Verification items for the finished model (mm, model axes). Give positions to 0.01 mm unless a question says otherwise; leave off trailing zeros. Order: outer loops, then holes, each group sorted by start corner. A loop starts at its lowest first (then second) coordinate and runs counter-clockwise, first axis right, second up.
(1) Sectioned sample at B-B on x = 20.5. Record the cut outline in (y, z), plus the area to 3 significant figures.
(2) Scan lines: L1, parallel to X at y = 1.7, z = -16; L2, parallel to Z at x = 57, y = -0.4; L3, parallel to X at y = -1.5, z = -10. Record each from-to range of solid material in increasing order.
(3) Gauge pin test, flat ends, axial feed: pin 1 (3 mm diameter, centred on y = 2, z = -9.5, fed in from +X); pin 2 (1.5 mm diameter, centred on y = 0.5, z = -13.5, fed in from +X); pin 3 (2.5 mm diameter, centred on y = 0.5, z = 15.5, fed in from +X); pin 4 (1.5 mm diameter, centred on y = 0.5, z = 17, fed in from -X). Record the tip position at first contact, or that the pin passes through.
(4) Sectioned sample at A-A on z = 5.5. Record the cut outline in (x, y), plus the area to 3 significant figures.
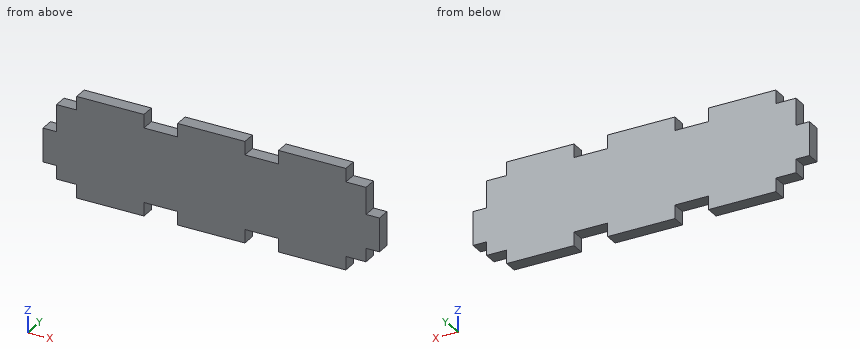
```python
from build123d import *

# Parameters (mm, degrees)
SKETCH1_W           = 127
SKETCH1_H           = 38.1
BOSS_EXTRUDE1_DEPTH = 2.54
SKETCH2_W           = 5.08
SKETCH2_H           = 10.16
SKETCH2_H_2         = 15.24
CUT_EXTRUDE1_DEPTH  = 5.08
SKETCH3_W           = 12.7
SKETCH3_H           = 5.08
CUT_EXTRUDE2_DEPTH  = 5.08
SKETCH4_W           = 12.7
SKETCH4_H           = 5.08
CUT_EXTRUDE4_DEPTH  = 5.08
LPATTERN1_COUNT     = 2
LPATTERN1_PITCH     = 38.1
SKETCH7_W           = 116.84
SKETCH7_H           = 5.08
CUT_EXTRUDE7_DEPTH  = 5.08
SKETCH8_W           = 25.4
SKETCH8_H           = 5.08
BOSS_EXTRUDE2_DEPTH = 5.08


with BuildPart() as part:
    # Sketch1 → Boss-Extrude1 (new body, symmetric)
    with BuildSketch(Plane(origin=(0, 0, 0), x_dir=(1, 0, 0), z_dir=(0, 1, 0))):
        Rectangle(SKETCH1_W, SKETCH1_H)
    extrude(amount=BOSS_EXTRUDE1_DEPTH, both=True)

    # Sketch2 → Cut-Extrude1 (cut)
    with BuildSketch(Plane(origin=(0, 2.54, 0), x_dir=(1, 0, 0), z_dir=(0, 1, 0))):
        with Locations((-60.96, 13.97)):
            Rectangle(SKETCH2_W, SKETCH2_H)
        with Locations((-60.96, -11.43)):
            Rectangle(SKETCH2_W, SKETCH2_H_2)
    cut_extrude1 = extrude(amount=-CUT_EXTRUDE1_DEPTH, mode=Mode.SUBTRACT)

    # Mirror1: Cut-Extrude1 across plane
    add(cut_extrude1.mirror(Plane(origin=(0, 0, 0), x_dir=(0, 0, 1), z_dir=(1, 0, 0))), mode=Mode.SUBTRACT)

    # Sketch3 → Cut-Extrude2 (cut)
    with BuildSketch(Plane(origin=(0, 2.54, 0), x_dir=(1, 0, 0), z_dir=(0, 1, 0))):
        with Locations((-57.15, -16.51)):
            Rectangle(SKETCH3_W, SKETCH3_H)
    cut_extrude2 = extrude(amount=-CUT_EXTRUDE2_DEPTH, mode=Mode.SUBTRACT)

    # Mirror2: Cut-Extrude2 across plane
    add(cut_extrude2.mirror(Plane(origin=(0, 0, 0), x_dir=(0, 0, 1), z_dir=(1, 0, 0))), mode=Mode.SUBTRACT)

    # Sketch4 → Cut-Extrude4 (cut)
    with BuildSketch(Plane(origin=(0, 2.54, 0), x_dir=(1, 0, 0), z_dir=(0, 1, 0))):
        with Locations((-19.05, -16.51)):
            Rectangle(SKETCH4_W, SKETCH4_H)
    cut_extrude4 = extrude(amount=-CUT_EXTRUDE4_DEPTH, mode=Mode.SUBTRACT)

    # LPattern1: Cut-Extrude4 ×2
    with Locations(*[(i * LPATTERN1_PITCH, 0, 0) for i in range(1, LPATTERN1_COUNT)]):
        add(cut_extrude4, mode=Mode.SUBTRACT)

    # Sketch7 → Cut-Extrude7 (cut)
    with BuildSketch(Plane(origin=(0, 2.54, 0), x_dir=(1, 0, 0), z_dir=(0, 1, 0))):
        with Locations((0, 16.51)):
            Rectangle(SKETCH7_W, SKETCH7_H)
    extrude(amount=-CUT_EXTRUDE7_DEPTH, mode=Mode.SUBTRACT)

    # Sketch8 → Boss-Extrude2 (add)
    with BuildSketch(Plane(origin=(0, 2.54, 0), x_dir=(1, 0, 0), z_dir=(0, 1, 0))):
        with Locations((-38.1, 16.51)):
            Rectangle(SKETCH8_W, SKETCH8_H)
        with Locations((0, 16.51)):
            Rectangle(SKETCH8_W, SKETCH8_H)
        with Locations((38.1, 16.51)):
            Rectangle(SKETCH8_W, SKETCH8_H)
    extrude(amount=-BOSS_EXTRUDE2_DEPTH)


solid = part.part
```
Ans:
1. outline: (-2.54, -13.97) - (2.54, -13.97) - (2.54, 13.97) - (-2.54, 13.97) - close
1. area: 142 mm2
2. L1: x = -50.8 to -25.4, -12.7 to 12.7, 25.4 to 50.8
2. L2: z = -13.97 to 13.97
2. L3: x = -58.42 to 58.42
3. pin 1: stops at x = 63.5
3. pin 2: stops at x = 58.42
3. pin 3: stops at x = 50.8
3. pin 4: stops at x = -50.8
4. outline: (-58.42, -2.54) - (58.42, -2.54) - (58.42, 2.54) - (-58.42, 2.54) - close
4. area: 594 mm2
